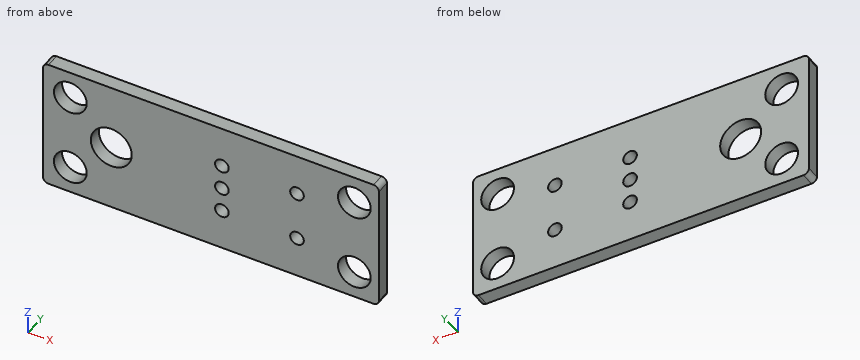
```python
from build123d import *

# Parameters (mm, degrees)
SKETCH1_W           = 123
SKETCH1_H           = 48
SKETCH1_R           = 6
SKETCH1_R_2         = 7.5
SKETCH1_R_3         = 2.5
BOSS_EXTRUDE1_DEPTH = 5
FILLET1_R           = 2


with BuildPart() as part:
    # Sketch1 → Boss-Extrude1 (new body)
    with BuildSketch(Plane(origin=(0, 0, 0), x_dir=(1, 0, 0), z_dir=(0, 1, 0))):
        with Locations((61.5, 24)):
            Rectangle(SKETCH1_W, SKETCH1_H)
        with Locations(Location((10, 10, 0), (0, 0, 270))):
            Circle(SKETCH1_R, mode=Mode.SUBTRACT)
        with Locations(Location((10, 38, 0), (0, 0, 270))):
            Circle(SKETCH1_R, mode=Mode.SUBTRACT)
        with Locations(Location((114, 38, 0), (0, 0, 270))):
            Circle(SKETCH1_R, mode=Mode.SUBTRACT)
        with Locations(Location((114, 10, 0), (0, 0, 270))):
            Circle(SKETCH1_R, mode=Mode.SUBTRACT)
        with Locations(Location((25, 24, 0), (0, 0, 270))):
            Circle(SKETCH1_R_2, mode=Mode.SUBTRACT)
        with Locations(Location((93, 15, 0), (0, 0, 270))):
            Circle(SKETCH1_R_3, mode=Mode.SUBTRACT)
        with Locations(Location((93, 33, 0), (0, 0, 270))):
            Circle(SKETCH1_R_3, mode=Mode.SUBTRACT)
        with Locations(Location((65.5, 15, 0), (0, 0, 270))):
            Circle(SKETCH1_R_3, mode=Mode.SUBTRACT)
        with Locations(Location((65.5, 24, 0), (0, 0, 270))):
            Circle(SKETCH1_R_3, mode=Mode.SUBTRACT)
        with Locations(Location((65.5, 33, 0), (0, 0, 270))):
            Circle(SKETCH1_R_3, mode=Mode.SUBTRACT)
    extrude(amount=BOSS_EXTRUDE1_DEPTH)

    # Fillet1
    fillet1_edges = [part.edges().sort_by_distance(p)[0] for p in [
        (0, 2.5, -48),
        (123, 2.5, -48),
        (123, 2.5, 0),
        (0, 2.5, 0),
    ]]
    fillet(fillet1_edges, radius=FILLET1_R)


solid = part.part
```
Model file for the job. Use its own axes, mm. Give positions to 0.01 mm unless a question says otherwise; leave off trailing zeros. Loops run counter-clockwise (first coordinate to the right, second up) from the corner with the lowest first, then second, coordinate; pieces in that order, holes last. Notation, with made-up numbers: (-33, -40) - (3, -40) arc R33 cw to (3, -1) - close; hole circle Ø8 at (15, 9.25). An arc over 180 degrees is marked (long way). One line per item, written item: value. Start each with the question number.
1. Slice it at D-D (y = 1.6). Give the number of separate pieces and of enclosed holes in the cut face, plus the area to 3 significant figures.
2. Probe L1, parallel to X at y = 1.6, z = -24; L2, parallel to X at y = 3.1, z = -38; L3, parallel to Z at x = 25.5, y = 0.65. List the from-to ranges inside material, lowest first. Write a range as from..to.
3. Slice it at A-A (x = 65.5). List the corners of the cut face in (y, z), plus the area to 3 significant figures.
4. Pin check, flat tip, straight feed: pin 1 (4 mm diameter, centred on x = 93, z = -15, fed in from +Y). Stop position of the tip, or through.
5. Slice it at B-B (z = -10). List the corners of the cut face in (x, y).
6. Slice it at C-C (x = 25). List the corners of the cut face in (y, z), plus the area to 3 significant figures.
Solution:
1. separate pieces: 1
1. enclosed holes: 10
1. area: 5,170 mm^2
2. L1: x = 0..17.5, 32.5..63, 68..123
2. L2: x = 0..4, 16..108, 120..123
2. L3: z = -48..-31.48, -16.52..0
3. outline: (0, -48) - (5, -48) - (5, -35.5) - (0, -35.5) - close; (0, -30.5) - (5, -30.5) - (5, -26.5) - (0, -26.5) - close; (0, -21.5) - (5, -21.5) - (5, -17.5) - (0, -17.5) - close; (0, -12.5) - (5, -12.5) - (5, 0) - (0, 0) - close
3. area: 165 mm^2
4. pin 1: passes through
5. outline: (0, 0) - (4, 0) - (4, 5) - (0, 5) - close; (16, 0) - (108, 0) - (108, 5) - (16, 5) - close; (120, 0) - (123, 0) - (123, 5) - (120, 5) - close
6. outline: (0, -48) - (5, -48) - (5, -31.5) - (0, -31.5) - close; (0, -16.5) - (5, -16.5) - (5, 0) - (0, 0) - close
6. area: 165 mm^2
